Build history of the part. All positions in model axes, mm. Give positions to 0.01 mm unless a question says otherwise; leave off trailing zeros. Loops run counter-clockwise (first coordinate to the right, second up) from the corner with the lowest first, then second, coordinate; pieces in that order, holes last. Notation, with made-up numbers: (-16.5, 67.25) -> (24.5, 67.25) arc R22 ccw to (24.5, 75.25) -> close; hole circle Ø7 at (59.25, 30). An arc over 180 degrees is marked (long way). Answer in a Markdown table with one row per item. Add a question column.
Autodesk Inventor part; units mm, degrees
ref_plane "YZ Plane" through (0, 0, 0) normal (1, 0, 0) x (0, 1, 0)
ref_plane "XZ Plane" through (0, 0, 0) normal (0, 1, 0) x (-1, 0, 0)
ref_plane "XY Plane" through (0, 0, 0) normal (0, 0, 1) x (1, 0, 0)
sketch "Sketch1" plane through (0, 0, 0) normal (0, 0, 1) x (1, 0, 0)
  line L0 (-20.75, -10) -> (20.75, -10)
  line L1 (20.75, -10) -> (20.75, 10)
  line L2 (20.75, 10) -> (-20.75, 10)
  line L3 (-20.75, 10) -> (-20.75, -10)
  line L4 (-20.75, -10) -> (20.75, 10) construction
  line L5 (20.75, -10) -> (-20.75, 10) construction
  circle A0 centre (-17.75, 4) radius 1.4
  circle A1 centre (-17.75, -4) radius 1.4
  point P0 (0, 0)
  dimension "d0" = 41.5
  dimension "d1" = 20
  dimension "d2" = 2.8
  dimension "d3" = 2.8
  dimension "d4" = 6
  dimension "d5" = 6
  dimension "d6" = 3
  dimension "d7" = 3
extrude "Extrusion1" add sketch "Sketch1" along normal blind 2
extrude "Extrusion2" add sketch "Sketch1" along normal blind 5.5 contours A0 | A1
fillet "Fillet1" radius 1 2 edges at (-19.15, -4, 5.5) (-19.15, 4, 5.5)
chamfer "Chamfer1" distance 0.8 angle 45 4 edges at (-20.75, 0, 2) (0, 10, 2) (0, -10, 2) (20.75, 0, 2)
sketch "Sketch2" plane through (0, 0, 2) normal (0, 0, 1) x (1, 0, 0)
  line L0 (20.75, -10) -> (20.75, 10)
  line L1 (20.75, -6.5) -> (-14.25, -6.5)
  line L2 (-14.25, -6.5) -> (-14.25, 6.5)
  line L3 (-14.25, 6.5) -> (20.75, 6.5)
  line L4 (20.75, 6.5) -> (20.75, -6.5)
  line L5 (20.75, 10) -> (-20.75, 10)
  line L6 (-20.75, -10) -> (20.75, -10)
  line L7 (-20.75, 10) -> (-20.75, -10)
  line L8 (20.75, 6.5) -> (13.25, 6.5)
  line L9 (13.25, 6.5) -> (13.25, -6.5)
  line L10 (13.25, -6.5) -> (20.75, -6.5)
  line L11 (20.75, -6.5) -> (20.75, 6.5)
  line L12 (13.25, -6.5) -> (3.25, -6.5)
  line L13 (3.25, -6.5) -> (3.25, 6.5)
  line L14 (3.25, 6.5) -> (13.25, 6.5)
  line L15 (13.25, 6.5) -> (13.25, -6.5)
  line L16 (-14.25, -6.5) -> (-14.75, -6.5)
  line L17 (-14.75, -6.5) -> (-14.75, 6)
  line L18 (-14.75, 6) -> (-14.25, 6)
  line L19 (-14.25, 6) -> (-14.25, -6.5)
  point P0 (0, 0)
  point P1 (20.75, 6.5)
  point P2 (3.25, -6.5)
  point P3 (-14.5, 6)
  point P4 (-14.5, 6)
  dimension "d16" = 3.5
  dimension "d17" = 3.5
  dimension "d18" = 6.5
  dimension "d19" = 7.5
  dimension "d20" = 10
  dimension "d23" = 0.5
extrude "Extrusion3" cut sketch "Sketch2" against normal blind 2.5 contours L1 L9 L3 L0 | L1 L2 L3 L13 | L16 L17 L18 L2
properties part number "Modules_cover"
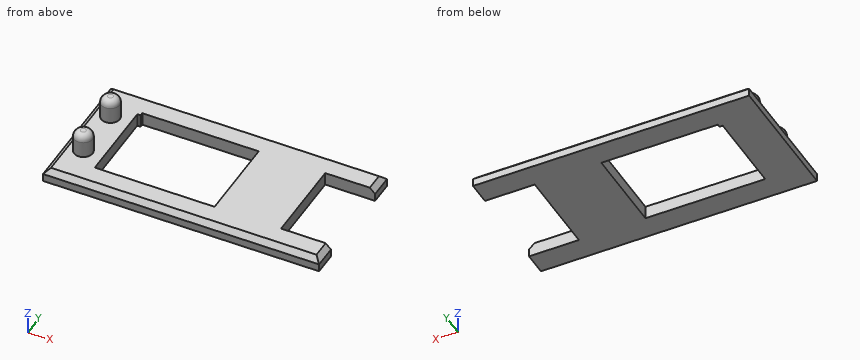
(1) Saw through at D-D, the plane z = 3.9. List the corners of the cut face in (x, y).
(2) Wall check: line 1 along Y through (x, z) = (13.5, 0.75); line 2 along Z through (x, y) = (9, -1.25); line 3 along X through (y, z) = (-5.25, 1.05). Give the ranges that are in metal, low to high. Write a range as from..to.
(3) Saw through at A-A, the plane x = -6.5. List the corners of the cut face in (y, z), then the cut area to 3 significant figures.
(4) Saw through at C-C, the plane x = 11.5. List the corners of the cut face in (y, z).
(5) Flat gauge pins, fed straight in: pin 1 Ø1 at (y, z) = (-0.5, 1) entering from +X; pin 2 Ø9 at (x, y) = (-6.5, -3.5) entering from +Z. Where does each tip first touch, or does it go through?
(6) Saw through at B-B, the plane y = -0.5. List the corners of the cut face in (x, z), then the cut area to 3 significant figures.
Worked answers:
| question | item | result |
|---|---|---|
| 1 | outline | circle Ø2.8 at (-17.75, -4); circle Ø2.8 at (-17.75, 4) |
| 2 | line 1 | -10..-6.5, 6.5..10 |
| 2 | line 2 | 0..2 |
| 2 | line 3 | -20.75..-14.75, 3.25..13.25 |
| 3 | outline | (-10, 0) -> (-6.5, 0) -> (-6.5, 2) -> (-9.2, 2) -> (-10, 1.2) -> close; (6.5, 0) -> (10, 0) -> (10, 1.2) -> (9.2, 2) -> (6.5, 2) -> close |
| 3 | area | 13.4 mm^2 |
| 4 | outline | (-10, 0) -> (10, 0) -> (10, 1.2) -> (9.2, 2) -> (-9.2, 2) -> (-10, 1.2) -> close |
| 5 | pin 1 | x = 13.25 |
| 5 | pin 2 | z = 2 |
| 6 | outline | (-20.75, 0) -> (-14.75, 0) -> (-14.75, 2) -> (-19.95, 2) -> (-20.75, 1.2) -> close; (3.25, 0) -> (13.25, 0) -> (13.25, 2) -> (3.25, 2) -> close |
| 6 | area | 31.7 mm^2 |
